Source: three-view drawing plus pictorial views. Frame: mm from the lowest corner of the part. A direction names the side the tool comes from. Give positions to 0.01 mm unless a question says otherwise; leave off trailing zeros. Order: outer loops, then holes, each group sorted by start corner. A loop starts at its lowest first (then second) coordinate and runs counter-clockwise, first axis right, second up.
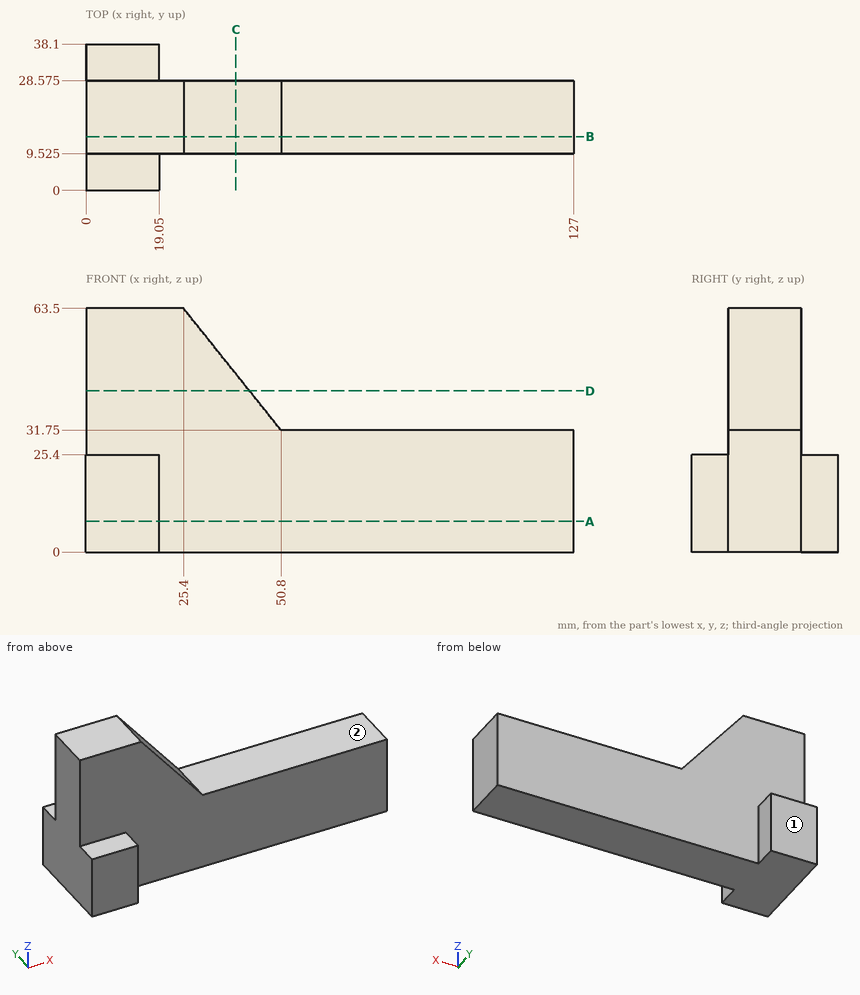
1) Section query A-A on z = 8. Output: boundary loops of the cut face in (x, y) (3 decimals).
Checks:
outline: (0, 0) - (19.05, 0) - (19.05, 9.525) - (127, 9.525) - (127, 28.575) - (19.05, 28.575) - (19.05, 38.1) - (0, 38.1) - close
2) Reachability of the marked faces 1 and 2 from +Z, -Z, +X, -X, +Y, -Y: full face, straight path, thin tool, end or side. Return the list, or none.
Checks:
face 1: +Z, -Z, +X, -X, +Y
face 2: +Z, +X, +Y, -Y
3) Section query D-D on z = 42. Output: boundary loops of the cut face in (x, y) (3 decimals).
Checks:
outline: (0, 9.525) - (42.6, 9.525) - (42.6, 28.575) - (0, 28.575) - close
4) Section query B-B on y = 14. Output: boundary loops of the cut face in (x, z), and give its area (3 significant figures).
Checks:
outline: (0, 0) - (127, 0) - (127, 31.75) - (50.8, 31.75) - (25.4, 63.5) - (0, 63.5) - close
area: 5,240 mm2
5) First-contact query: pin 1 Ø1 at (x, z) = (79.5, 16.5) entering from -Y (3 decimals); pin 2 Ø3 at (x, y) = (10, 6) entering from +Z; pin 3 Ø8 at (x, z) = (35, 16.5) entering from +Y (3 decimals). Flat tips, straight axial feed; report the tip coordinate or a pass-through.
Checks:
pin 1: stops at y = 9.525
pin 2: stops at z = 25.4
pin 3: stops at y = 28.575
6) Section query C-C on x = 39. Output: boundary loops of the cut face in (y, z) (3 decimals).
Checks:
outline: (9.525, 0) - (28.575, 0) - (28.575, 46.5) - (9.525, 46.5) - close
7) Ray query, L1, parallel to Y at x = 38, z = 30.5 (3 decimals); L2, parallel to Z at x = 7, y = 34; L3, parallel to Z at x = 119, y = 13.5. Return the intervals inside material, ascending.
Checks:
L1: y = 9.525 to 28.575
L2: z = 0 to 25.4
L3: z = 0 to 31.75
